from build123d import *

# Parameters (mm, degrees)
F0_R     = 53.5
F0_R_2   = 51.5
F1_DEPTH = 30
F2_T     = -1.5
F3_R     = 32
F4_DEPTH = 25


with BuildPart() as f1:
    # F0 (on Front) → F1 (new body)
    with BuildSketch(Plane.XZ):
        Circle(F0_R)
        Circle(F0_R_2, mode=Mode.SUBTRACT)
        Circle(F0_R_2)
    extrude(amount=F1_DEPTH)

    # F2
    f2_openings = [f1.faces().sort_by_distance(p)[0] for p in [
        (0, -30, 0),
    ]]
    offset(amount=F2_T, openings=f2_openings)

    # F3 (on face) → F4 (cut)
    with BuildSketch(Plane.XZ.offset(1.5)):
        Circle(F3_R)
    extrude(amount=-F4_DEPTH, mode=Mode.SUBTRACT)


solid = f1.part
Part model, mm, in its own coordinate system. A direction names the side the tool comes from. Give positions to 0.01 mm unless a question says otherwise; leave off trailing zeros. Order: outer loops, then holes, each group sorted by start corner. A loop starts at its lowest first (then second) coordinate and runs counter-clockwise, first axis right, second up. Notation, with made-up numbers: (88, -21.75) - (108, -21.75) arc R29 ccw to (108, 8.25) - close; hole circle Ø2 at (-21, -37.5). An arc over 180 degrees is marked (long way). One line per question, with ' | ' between items.
1. Band-saw the part on D-D on x = -41. List the corners of the cut face in (y, z), then the cut area to 3 significant figures.
Filled in:
outline: (-30, -34.37) - (0, -34.37) - (0, 34.37) - (-30, 34.37) - (-30, 31.98) - (-1.5, 31.98) - (-1.5, -31.98) - (-30, -31.98) - close | area: 239 mm²
2. Band-saw the part on B-B on z = 0. List the corners of the cut face in (x, y), then the cut area to 3 significant figures.
Filled in:
outline: (-53.5, -30) - (-52, -30) - (-52, -1.5) - (-32, -1.5) - (-32, 0) - (-53.5, 0) - close; (32, -1.5) - (52, -1.5) - (52, -30) - (53.5, -30) - (53.5, 0) - (32, 0) - close | area: 150 mm²
3. Band-saw the part on C-C on z = -44. List the corners of the cut face in (x, y).
Filled in:
outline: (-30.43, -30) - (-27.71, -30) - (-27.71, -1.5) - (27.71, -1.5) - (27.71, -30) - (30.43, -30) - (30.43, 0) - (-30.43, 0) - close
4. Pull direction Z, two halves, no side cores. Call faces 3 (the face through (-41.265, -15.55, -31.641)), 4 (the face through (23, 0, -23)), 5 (the face through (-11.598, -14.79, -52.228)): +Z half, -Z half, draft (parallel to the pull), parting line (faces both ways), or undercut.
Filled in:
face 3: undercut | face 4: draft | face 5: parting line
5. Band-saw the part on A-A on x = 0. List the corners of the cut face in (y, z), then the cut area to 3 significant figures.
Filled in:
outline: (-30, -53.5) - (0, -53.5) - (0, -32) - (-1.5, -32) - (-1.5, -52) - (-30, -52) - close; (-30, 52) - (-1.5, 52) - (-1.5, 32) - (0, 32) - (0, 53.5) - (-30, 53.5) - close | area: 150 mm²
6. Which spindle directions (+Z, -Z, +X, -X, +Y, -Y) get a long thin tool onto all of the face, cutting with end or side? Do faces 1 (the face through (-44, -30, 28)), 2 (the face through (22, -1.5, 24)). Say none if no direction does.
Filled in:
face 1: +Z, -Z, +X, -X, -Y | face 2: -Y
7. Drill centre lines: probe 1 along Z at (x, y) = (0, -21.75); probe 2 along Z at (x, y) = (0, -0.95); probe 3 along Y at (x, z) = (39, 30.5). Where is each one in solid material? Low to high.
Filled in:
probe 1: -53.5 to -52, 52 to 53.5 | probe 2: -53.5 to -32, 32 to 53.5 | probe 3: -1.5 to 0
8. Drop flat-ended pins along their axis: P1, Ø12, axis at y = -13, z = 13, coming from the -X side; P2, Ø8, axis at x = -15, y = -15, coming from the -Z side; P3, Ø1, axis at x = -3.5, y = -8.5, coming from the -Z side. Give the stop position or say it passes through.
Filled in:
P1: x = -53.04 | P2: z = -52.36 | P3: z = -53.42
